Here's how the part is built. I have some questions about the finished solid (model axes, mm). Face numbers are marked on the shaded views. A direction names the side the tool comes from. Round coordinates to 2 decimals unless told otherwise and drop trailing zeros. Loops run counter-clockwise (first coordinate to the right, second up) from the corner with the lowest first, then second, coordinate; pieces in that order, holes last. Notation, with made-up numbers: M 9,-26 L 38,-26 A30 cw 38,0 Z; hole C 86,54.25 d5. An arc over 180 degrees is marked long. Answer as a JSON object with one key per item and string values.
from build123d import *


with BuildPart() as part:
    # Çizim1 → Döndür1 (revolve)
    with BuildSketch(Plane(origin=(0, 0, 0), x_dir=(1, 0, 0), z_dir=(0, 1, 0)), mode=Mode.PRIVATE) as d_nd_r1_sk:
        with BuildLine():
            Line((12.781543507, 13.383116119), (-2.50303312, 13.383116119))
            ThreePointArc((-2.50303312, 13.383116119), (-2.501361875, 13.293526957), (-2.506133274, 13.204049335))
            Line((-2.506133274, 13.204049335), (-2.506133274, 9.63773694))
            Line((-2.506133274, 9.63773694), (0, 9.63773694))
            Line((0, 9.63773694), (0, 3.705))
            Line((0, 3.705), (4.808638309, 3.705))
            ThreePointArc((4.808638309, 3.705), (5.009621244, 3.664180843), (5.185678757, 3.558994837))
            ThreePointArc((5.185678757, 3.558994837), (7.965698705, 8.014106646), (12.465543511, 10.721121396))
            ThreePointArc((12.465543511, 10.721121396), (12.633558311, 10.915283437), (12.780786925, 11.125644095))
            Line((12.780786925, 11.125644095), (12.781543507, 13.383116119))
        make_face()
    revolve(d_nd_r1_sk.sketch.rotate(Axis((0, 0, 0), (1, 0, 0)), 180), axis=Axis((0, 0, 0), (1, 0, 0)))

    # Çizim2 → Kes-Döndür3 (revolve, cut)
    with BuildSketch(Plane.ZY.offset(-12.773866726)):
        with BuildLine():
            Line((13.385193973, 0), (-13.385193973, 0))
            Line((-13.385193973, 0), (-16.077753665, 0))
            Line((-16.077753665, 0), (-16.077753665, 10.025014185))
            Line((-16.077753665, 10.025014185), (-8.869188704, 10.025014185))
            add(Edge.make_bspline(
                [(-4.830106972, 10.024782411), (-6.17646756, 10.024842425), (-7.522828137, 10.024922597), (-8.869188704, 10.025014185)],
                knots=[0.002442016, 0.002442016, 0.002442016, 0.002442016, 0.006481098, 0.006481098, 0.006481098, 0.006481098], degree=3))
            add(Edge.make_bspline(
                [(-4.065295391, 9.922720168), (-4.309706946, 9.966250241), (-4.566541382, 9.998257381), (-4.830106972, 10.024782411)],
                knots=[0, 0, 0, 0, 1, 1, 1, 1], degree=3))
            ThreePointArc((-4.065295391, 9.922720168), (0, 10.723199249), (4.065295391, 9.922720168))
            add(Edge.make_bspline(
                [(4.830106972, 10.024782411), (4.567249442, 9.99832864), (4.310513413, 9.966393874), (4.065295391, 9.922720168)],
                knots=[0, 0, 0, 0, 1, 1, 1, 1], degree=3))
            add(Edge.make_bspline(
                [(8.869188704, 10.025014185), (7.522828137, 10.024922597), (6.17646756, 10.024842425), (4.830106972, 10.024782411)],
                knots=[-0.01125728, -0.01125728, -0.01125728, -0.01125728, -0.007218198, -0.007218198, -0.007218198, -0.007218198], degree=3))
            Line((8.869188704, 10.025014185), (15.518432284, 10.025014185))
            Line((15.518432284, 10.025014185), (15.518432284, 0))
            Line((15.518432284, 0), (13.385193973, 0))
        make_face()
    revolve(axis=Axis((12.773866726, 0, -16.077753665), (0, 0, 1)), mode=Mode.SUBTRACT)


solid = part.part
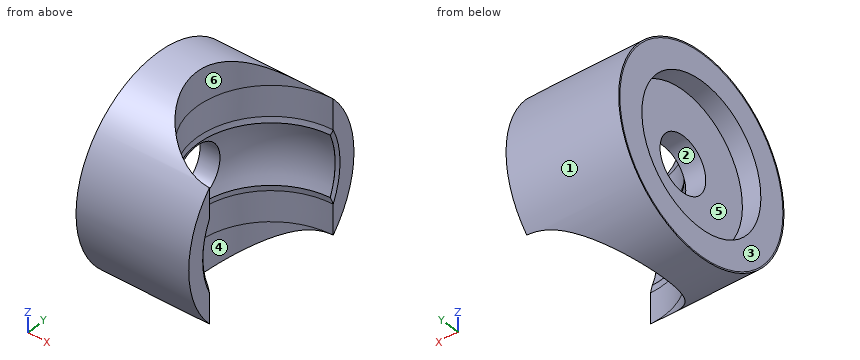
Item 1: For the marked faces 4, 5 and 6, which set-ups out of +Z, -Z, +X, -X, +Y, -Y let a thin tool reach every point of the face, with its end or its side?
Solution:
{"face 4": "-Z, +X", "face 5": "-X", "face 6": "+Z, +X"}
Item 2: If I drill on L1, parallel to Y at x = 0.75, z = 0 (3 decimals); L2, parallel to Y at x = 6, z = -4; L3, parallel to Z at x = -1.5, y = 5, over which ranges is the centre line in solid material (lowest first)? Write a range as from..to.
Solution:
{"L1": "y = -13.383..-3.705, 3.705..13.383", "L2": "y = -12.77..-7.29, 7.29..12.77", "L3": "z = -12.41..-8.24, 8.24..12.41"}
Item 3: For P1, Ø4, axis at y = 5.5, z = -6.5, coming from the -X side; P2, Ø15.5, axis at y = 0, z = 0.5, coming from the -X side; P3, Ø2, axis at x = 0, y = -6, coming from the +Z side; P4, Ø4, axis at x = 10, y = 7, coming from the -Z side, each with a flat end and sliding along its axis, tell me the tip position at first contact or that it passes through.
Solution:
{"P1": "stops at x = -2.51", "P2": "stops at x = 0", "P3": "stops at z = 12.41", "P4": "passes through"}
Item 4: I want a section at A-A on x = 0.75. List the corners of the cut face in (y, z) for me (3 decimals).
Solution:
{"outline": "C 0,0 d26.766; hole C 0,0 d7.41"}
Item 5: We'd pull the mould along Z, two halves only. Please class the marked faces 1, 2 and 3: +Z half, -Z half, draft (parallel to the pull), parting line (faces both ways), or undercut.
Solution:
{"face 1": "parting line", "face 2": "undercut", "face 3": "draft"}
